from build123d import *

# Parameters (mm, degrees)
F0_W     = 180
F0_H     = 130
F0_W_2   = 10
F0_H_2   = 100
F1_DEPTH = 1.5


with BuildPart() as f1:
    # F0 (on Top) → F1 (new body)
    with BuildSketch(Plane.XY):
        Rectangle(F0_W, F0_H)
        with Locations((-70, 0)):
            Rectangle(F0_W_2, F0_H_2, mode=Mode.SUBTRACT)
        with Locations((-50, 0)):
            Rectangle(F0_W_2, F0_H_2, mode=Mode.SUBTRACT)
        with Locations((-30, 0)):
            Rectangle(F0_W_2, F0_H_2, mode=Mode.SUBTRACT)
        with Locations((-10, 0)):
            Rectangle(F0_W_2, F0_H_2, mode=Mode.SUBTRACT)
        with Locations((10, 0)):
            Rectangle(F0_W_2, F0_H_2, mode=Mode.SUBTRACT)
        with Locations((30, 0)):
            Rectangle(F0_W_2, F0_H_2, mode=Mode.SUBTRACT)
        with Locations((50, 0)):
            Rectangle(F0_W_2, F0_H_2, mode=Mode.SUBTRACT)
        with Locations((70, 0)):
            Rectangle(F0_W_2, F0_H_2, mode=Mode.SUBTRACT)
    extrude(amount=F1_DEPTH)


solid = f1.part
Can you work these out from the model? Positions are in its coordinate system, mm. Round coordinates to 2 decimals unless told otherwise and drop trailing zeros. Order: outer loops, then holes, each group sorted by start corner. A loop starts at its lowest first (then second) coordinate and runs counter-clockwise, first axis right, second up. Notation, with made-up numbers: (58.5, 37) - (88.5, 37) arc R23 cw to (88.5, 60) - close; hole circle Ø3 at (-13, -16). An arc over 180 degrees is marked (long way). Answer in a Markdown table with one row per item.
(1) Suppose I cut it at B-B, the plane z = 0.6. Count the separate pieces of the cut face and the enclosed holes in it, plus the area to 3 significant figures.
From the geometry:
| item | result |
|---|---|
| separate pieces | 1 |
| enclosed holes | 8 |
| area | 15,400 mm2 |
(2) Please list where this line runs through material, in increasing order: L1, parallel to Y at x = 26, z = 1.3. Write a range as from..to.
From the geometry:
| item | result |
|---|---|
| L1 | y = -65..-50, 50..65 |
(3) Suppose I cut it at A-A, the plane x = 11. Please give me the cut outline in (y, z).
From the geometry:
| item | result |
|---|---|
| outline | (-65, 0) - (-50, 0) - (-50, 1.5) - (-65, 1.5) - close; (50, 0) - (65, 0) - (65, 1.5) - (50, 1.5) - close |
